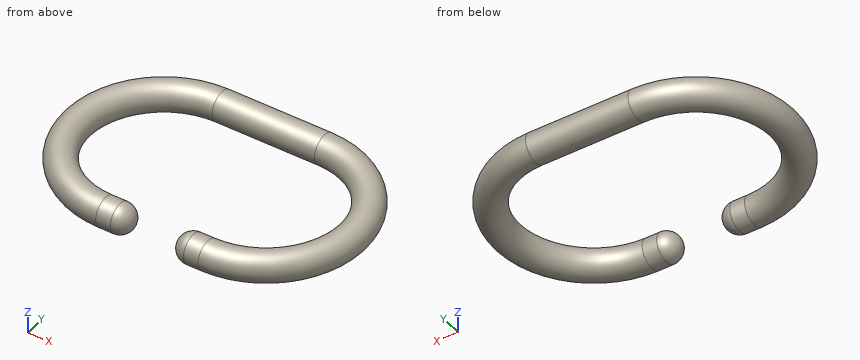
```python
from build123d import *

# Parameters (mm, degrees)
F2_R = 3
F4_R = 3


with BuildPart() as f3:
    # F3: sweep along a path in F0
    with BuildLine(Plane.XY) as f3_path:
        Line((-4.5, -17.5), (-10.5, -17.5))
        ThreePointArc((-10.5, -17.5), (-28, 0), (-10.5, 17.5))
        Line((-10.5, 17.5), (0, 17.5))
        Line((0, 17.5), (10.5, 17.5))
        ThreePointArc((10.5, 17.5), (28, 0), (10.5, -17.5))
        Line((10.5, -17.5), (4.5, -17.5))
    # F2 (on plane+point) → F3 (sweep)
    with BuildSketch(Plane.YZ.offset(-4.5)):
        with Locations((-17.5, 0)):
            Circle(F2_R)
    sweep(path=f3_path.line)

    # F4
    f4_edges = [f3.edges().sort_by_distance(p)[0] for p in [
        (-4.5, -20.5, 0),
        (4.5, -20.5, 0),
    ]]
    fillet(f4_edges, radius=F4_R)


solid = f3.part
```
Verification items for the finished model (mm, model axes). Coordinates: 2 decimals unless noted, no trailing zeros. Order: outer loops, then holes, each group sorted by start corner. A loop starts at its lowest first (then second) coordinate and runs counter-clockwise, first axis right, second up. Notation, with made-up numbers: (-20, 16) -> (-9, 16) arc R34 cw to (-9, 46) -> close; hole circle Ø10 at (63, 38). An arc over 180 degrees is marked (long way). Answer as CSV lines item,"result". Start each with the question number.
1) Cross-section at B-B, the plane x = -1. Record the boundary of the cut face in (y, z).
2) Cross-section at A-A, the plane z = 0. Record the boundary of the cut face in (x, y), then the cut area to 3 significant figures.
3) Gauge pin test, flat ends, axial feed: pin 1 Ø3 at (x, z) = (18, -1.5) entering from +Y; pin 2 Ø2 at (x, z) = (-6.5, -0.5) entering from -Y; pin 3 Ø8 at (x, y) = (6.5, 12) entering from +Z. Record the tip position at first contact, or that the pin passes through.
4) Material ranges on L1, parallel to Y at x = -9.5, z = 0.25; L2, parallel to Y at x = -16, z = -1; L3, parallel to X at y = -3.5, z = 1, recorded low to high. Write a range as [from, to].
Conclusion:
1,outline,"circle Ø6 at (17.5, 0)"
2,outline,"(-10.5, -20.5) -> (-7.5, -20.5) arc R3 ccw to (-7.5, -14.5) -> (-10.5, -14.5) arc R14.5 cw to (-10.5, 14.5) -> (10.5, 14.5) arc R14.5 cw to (10.5, -14.5) -> (7.5, -14.5) arc R3 ccw to (7.5, -20.5) -> (10.5, -20.5) arc R20.5 ccw to (10.5, 20.5) -> (-10.5, 20.5) arc R20.5 ccw to start"
2,area,"850 mm²"
3,pin 1,"stops at y = 19.44"
3,pin 2,"stops at y = -20.5"
3,pin 3,"stops at z = 2.6"
4,L1,"y = [-20.49, -14.51], [14.51, 20.49]"
4,L2,"y = [-19.57, -13.6], [13.6, 19.57]"
4,L3,"x = [-30.52, -24.75], [24.75, 30.52]"
